from build123d import *

# Parameters (mm, degrees)
SKETCH3_R          = 1.5
CUT_EXTRUDE1_DEPTH = 3


with BuildPart() as part:
    # Sketch2 → Revolve1 (revolve)
    with BuildSketch(Plane.XY, mode=Mode.PRIVATE) as revolve1_sk:
        Polygon((0, 0), (0, 12.5), (60.5, 12.5), (60.5, 3.400000058), (63.5, 3.400000058), (63.5, 2), (73.2, 2), (73.2, 0), align=None)
    revolve(revolve1_sk.sketch.rotate(Axis((73.2, 0, 0), (-1, 0, 0)), 90), axis=Axis((73.2, 0, 0), (-1, 0, 0)))

    # Sketch3 → Cut-Extrude1 (cut)
    with BuildSketch(Plane(origin=(60.5, 0, 0), x_dir=(0, 0, -1), z_dir=(1, 0, 0))):
        with Locations((8.15, 0)):
            Circle(SKETCH3_R)
        with Locations((-8.15, 0)):
            Circle(SKETCH3_R)
    extrude(amount=-CUT_EXTRUDE1_DEPTH, mode=Mode.SUBTRACT)


solid = part.part
Build history of the part. All positions in model axes, mm. A direction names the side the tool comes from. Give positions to 0.01 mm unless a question says otherwise; leave off trailing zeros. Order: outer loops, then holes, each group sorted by start corner. A loop starts at its lowest first (then second) coordinate and runs counter-clockwise, first axis right, second up. Notation, with made-up numbers: M 75,-29 L 125,-29 A18 ccw 125,-3 Z; hole C 85,27.25 d8. An arc over 180 degrees is marked long. Put each result on its own line as item: value.
Item 1: Slice it at B-B, the plane z = 0. Write the cut outline in (x, y).
From the geometry:
outline: M 0,-12.5 L 60.5,-12.5 L 60.5,-3.4 L 63.5,-3.4 L 63.5,-2 L 73.2,-2 L 73.2,2 L 63.5,2 L 63.5,3.4 L 60.5,3.4 L 60.5,12.5 L 0,12.5 Z
Item 2: Probe line 1 (X direction, y = 10.25, z = 5.5); line 2 (Z direction, x = 24, y = 0.25); line 3 (Y direction, x = 59.45, z = -8.15). List the from-to ranges inside material, lowest first. Write a range as [from, to].
From the geometry:
line 1: x = [0, 60.5]
line 2: z = [-12.5, 12.5]
line 3: y = [-9.48, -1.5], [1.5, 9.48]
Item 3: Slice it at A-A, the plane y = 0. Write the cut outline in (x, z), plus the area to 3 significant figures.
From the geometry:
outline: M 0,-12.5 L 60.5,-12.5 L 60.5,-9.65 L 57.5,-9.65 L 57.5,-6.65 L 60.5,-6.65 L 60.5,-3.4 L 63.5,-3.4 L 63.5,-2 L 73.2,-2 L 73.2,2 L 63.5,2 L 63.5,3.4 L 60.5,3.4 L 60.5,6.65 L 57.5,6.65 L 57.5,9.65 L 60.5,9.65 L 60.5,12.5 L 0,12.5 Z
area: 1,550 mm2
Item 4: Slice it at D-D, the plane z = 8.15. Write the cut outline in (x, y).
From the geometry:
outline: M 0,-9.48 L 60.5,-9.48 L 60.5,-1.5 L 57.5,-1.5 L 57.5,1.5 L 60.5,1.5 L 60.5,9.48 L 0,9.48 Z
Item 5: 3-axis set-ups, long thin cutter, end or side, ignore diameter. For faces 5 (the flat face through (60.5, 3, -3)), 6 (the flat face through (0, 0, 0)): which of +Z, -Z, +X, -X, +Y, -Y reach the whole face in a straight line?
From the geometry:
face 5: +X
face 6: +Z, -Z, -X, +Y, -Y
Item 6: Two-plate mould, pull along Y, no slides. Class faces 1 (the cylindrical face through (68, 2, 0)), 2 (the flat face through (73.2, 0, 0)), 3 (the flat face through (57.5, 0, -8)), 4 (the cylindrical face through (59.021, -0.575, 6.764)): +Y half, -Y half, draft (parallel to the pull), parting line (faces both ways), or undercut.
From the geometry:
face 1: parting line
face 2: draft
face 3: undercut
face 4: undercut
Item 7: Flat gauge pins, fed straight in: pin 1 Ø1 at (x, z) = (18, 6.5) entering from -Y; pin 2 Ø2.5 at (y, z) = (0.5, -7.5) entering from +X; pin 3 Ø0.9 at (y, z) = (-0.5, 8) entering from +X. Where does each tip first touch, or does it go through?
From the geometry:
pin 1: stops at y = -10.97
pin 2: stops at x = 60.5
pin 3: stops at x = 57.5
Item 8: Slice it at C-C, the plane x = 42.5. Write the cut outline in (y, z).
From the geometry:
outline: C 0,0 d25
